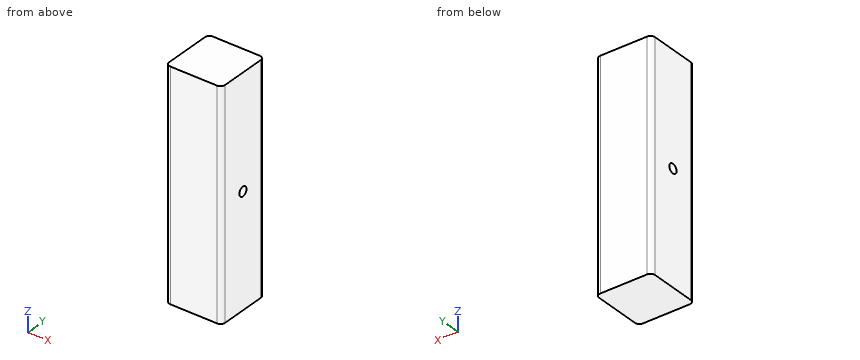
from build123d import *

# Parameters (mm, degrees)
SKETCH1_W           = 38.1
SKETCH1_H           = 38.1
BOSS_EXTRUDE1_DEPTH = 152.4
FILLET1_R           = 3.175
SKETCH2_R           = 3.175
CUT_EXTRUDE1_DEPTH  = 159.241184589


with BuildPart() as part:
    # Sketch1 → Boss-Extrude1 (new body)
    with BuildSketch(Plane.XY):
        Rectangle(SKETCH1_W, SKETCH1_H)
    extrude(amount=BOSS_EXTRUDE1_DEPTH)

    # Fillet1
    fillet1_edges = [part.edges().sort_by_distance(p)[0] for p in [
        (19.05, -19.05, 76.2),
        (-19.05, -19.05, 76.2),
        (-19.05, 19.05, 76.2),
        (19.05, 19.05, 76.2),
    ]]
    fillet(fillet1_edges, radius=FILLET1_R)

    # Sketch2 → Cut-Extrude1 (cut, through all)
    with BuildSketch(Plane.ZY.offset(19.05)):
        with Locations((76.2, 0)):
            Circle(SKETCH2_R)
    extrude(amount=-CUT_EXTRUDE1_DEPTH, mode=Mode.SUBTRACT)


solid = part.part
Could you check a few things on this model? Use its own coordinates, in mm. Round coordinates to 2 decimals unless told otherwise and drop trailing zeros. Order: outer loops, then holes, each group sorted by start corner. A loop starts at its lowest first (then second) coordinate and runs counter-clockwise, first axis right, second up.
(1) Imagine slicing it at B-B (z = 76.2). Write out the boundary of the cut face in (x, y) (3 decimals), plus the area to 3 significant figures.
Response values:
outline: (-19.05, -15.875) arc R3.175 ccw to (-15.875, -19.05) - (15.875, -19.05) arc R3.175 ccw to (19.05, -15.875) - (19.05, -3.175) - (-19.05, -3.175) - close; (-19.05, 3.175) - (19.05, 3.175) - (19.05, 15.875) arc R3.175 ccw to (15.875, 19.05) - (-15.875, 19.05) arc R3.175 ccw to (-19.05, 15.875) - close
area: 1,200 mm2
(2) Please list where these lines run through material, in increasing order: line 1 along Y through (x, z) = (-3.5, 76.2) (3 decimals); line 2 along Z through (x, y) = (-16, 1); line 3 along Y through (x, z) = (16, 9).
Response values:
line 1: y = -19.05 to -3.175, 3.175 to 19.05
line 2: z = 0 to 73.19, 79.21 to 152.4
line 3: y = -19.05 to 19.05
(3) Imagine slicing it at A-A (y = 0). Write out the boundary of the cut face in (x, z) (3 decimals), plus the area to 3 significant figures.
Response values:
outline: (-19.05, 0) - (19.05, 0) - (19.05, 73.025) - (-19.05, 73.025) - close; (-19.05, 79.375) - (19.05, 79.375) - (19.05, 152.4) - (-19.05, 152.4) - close
area: 5,560 mm2
